For this review, take the finished solid that the model builds, in its own axes (mm). Face numbers are marked on the shaded views. Round coordinates to 2 decimals unless told otherwise and drop trailing zeros. Write each loop counter-clockwise with the first axis right and the second up, starting at its lowest first coordinate (ties: lowest second). Pieces come first, ordered by that corner, then holes. Notation, with made-up numbers: (36, -29) -> (63, -29) arc R21 ccw to (63, -7) -> close; hole circle Ø2 at (15.25, 18.5). An arc over 180 degrees is marked (long way). Answer in a Markdown table with one row per item. Add a question column.
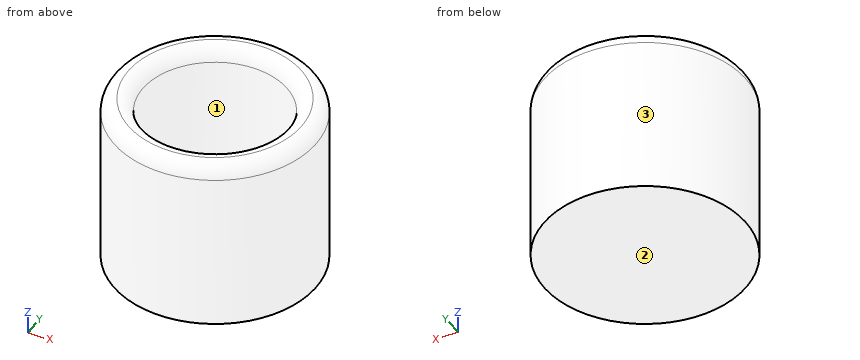
```python
from build123d import *

# Parameters (mm, degrees)
F2_R     = 70
F3_DEPTH = 20
F4_R     = 70
F4_R_2   = 50
F5_DEPTH = 100
F6_R     = 9.99999


# Not quite as in the source:
# - a fillet or chamfer is up to 0.001 mm smaller than in the source, because OpenCascade refuses the exact size


with BuildPart() as f3:
    # F2 (on Top) → F3 (new body)
    with BuildSketch(Plane.XY):
        Circle(F2_R)
    extrude(amount=F3_DEPTH)

    # F4 (on face) → F5 (join)
    with BuildSketch(Plane.XY.offset(20)):
        Circle(F4_R)
        Circle(F4_R_2, mode=Mode.SUBTRACT)
    extrude(amount=F5_DEPTH)

    # F6 (radius 10 in the source; OpenCascade refuses exactly that, so slightly less here)
    f6_edges = [f3.edges().sort_by_distance(p)[0] for p in [
        (-50, 0, 120),
        (-70, 0, 120),
    ]]
    fillet(f6_edges, radius=F6_R)


solid = f3.part
```
1. Clearance check with flat-ended pins moving along their axes: pin 1 Ø12 at (y, z) = (21, 91) entering from +X; pin 2 Ø6 at (y, z) = (45, 96) entering from -X; pin 3 Ø10 at (x, z) = (-44, 70) entering from +Y. State where each tip first meets the part, or that it passes through.
2. We need section C-C (z = 50.5). Write out the cut boundary in (x, y), plus the area to 3 significant figures.
3. We need section D-D (z = 17.5). Write out the cut boundary in (x, y), plus the area to 3 significant figures.
4. The part is to be moulded in two halves that separate along X. For the marked faces 1, 2 and 3, say which applies: pulls with the +X half, pulls with the -X half, needs draft (parallel to the pull), parting line crosses it, or undercut.
5. For L1, parallel to Y at x = 0, z = 76; L2, parallel to Z at x = 5.5, y = -46; L3, parallel to Y at x = -39, z = 64, list the stretches that pass through material, from the lowest coordinate up. Write a range as [from, to].
Response:
| question | item | result |
|---|---|---|
| 1 | pin 1 | x = 68.37 |
| 1 | pin 2 | x = -56 |
| 1 | pin 3 | y = 58.13 |
| 2 | outline | circle Ø140 at (0, 0); hole circle Ø100 at (0, 0) |
| 2 | area | 7,540 mm2 |
| 3 | outline | circle Ø140 at (0, 0) |
| 3 | area | 15,400 mm2 |
| 4 | face 1 | undercut |
| 4 | face 2 | needs draft |
| 4 | face 3 | parting line crosses it |
| 5 | L1 | [-70, -50], [50, 70] |
| 5 | L2 | [0, 20] |
| 5 | L3 | [-58.13, -31.29], [31.29, 58.13] |
